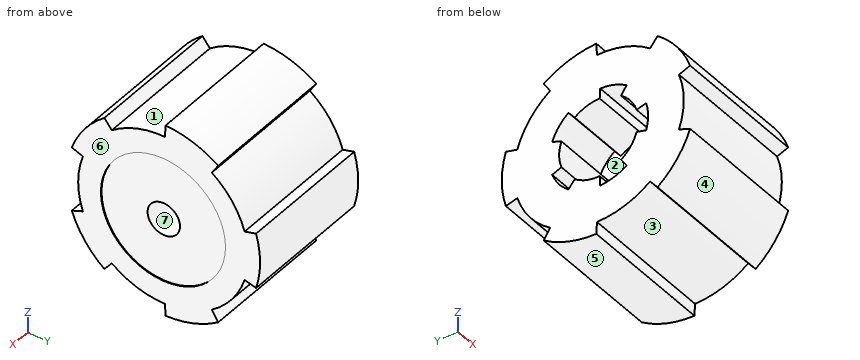
from build123d import *

# Parameters (mm, degrees)
SKETCH4_R                 = 21.5
BOSS_EXTRUDE1_DEPTH       = 34
BOSS_EXTRUDE2_DEPTH       = 34
CIRPATTERN1_COUNT         = 5
SKETCH7_R                 = 10
SHORTSHAFT_KEY1_DEPTH     = 16
SHORTSHAFT_KEY2_DEPTH     = 16
SHORTSHAFT_KEY_PATT_COUNT = 5
SKETCH10_R                = 15.75
PULLEYINDENTATION_DEPTH   = 0.2
SKETCH11_R                = 4.1
METAL_SHAFT_HOLE_DEPTH    = 14.5


with BuildPart() as part:
    # Sketch4 → Boss-Extrude1 (new body)
    with BuildSketch(Plane(origin=(0, 0, 0), x_dir=(0, 0, -1), z_dir=(1, 0, 0))):
        Circle(SKETCH4_R)
    extrude(amount=-BOSS_EXTRUDE1_DEPTH)

    # Sketch5 → Boss-Extrude2 (add)
    with BuildSketch(Plane(origin=(0, 0, 0), x_dir=(0, 0, -1), z_dir=(1, 0, 0))):
        with BuildLine():
            Line((-6.223542865, 20.579541156), (-7, 23.477318635))
            ThreePointArc((-7, 23.477318635), (0, 24.498663031), (7, 23.477318635))
            Line((7, 23.477318635), (6.223542865, 20.579541156))
            ThreePointArc((6.223542865, 20.579541156), (0, 21.5), (-6.223542865, 20.579541156))
        make_face()
    boss_extrude2 = extrude(amount=-BOSS_EXTRUDE2_DEPTH)

    # CirPattern1: Boss-Extrude2 ×5 about axis
    cirpattern1_axis = Axis((0, 0, 0), (1, 0, 0))
    for i in range(1, CIRPATTERN1_COUNT):
        add(boss_extrude2.rotate(cirpattern1_axis, i * 360 / CIRPATTERN1_COUNT))

    # Sketch7 → ShortShaft Key1 (cut)
    with BuildSketch(Plane.ZY.offset(34)):
        Circle(SKETCH7_R)
    extrude(amount=-SHORTSHAFT_KEY1_DEPTH, mode=Mode.SUBTRACT)

    # Sketch8 → ShortShaft Key2 (cut)
    with BuildSketch(Plane.ZY.offset(34)):
        with BuildLine():
            Line((-7.941654077, 6.077016581), (-9.88451898, 7.650317559))
            ThreePointArc((-9.88451898, 7.650317559), (-7.346870668, 10.11209996), (-4.22140002, 11.764814325))
            Line((-4.22140002, 11.764814325), (-3.325480146, 9.430863258))
            ThreePointArc((-3.325480146, 9.430863258), (-5.877852523, 8.090169944), (-7.941654077, 6.077016581))
        make_face()
    shortshaft_key2 = extrude(amount=-SHORTSHAFT_KEY2_DEPTH, mode=Mode.SUBTRACT)

    # ShortShaft Key Patt: ShortShaft Key2 ×5 about axis
    shortshaft_key_patt_axis = Axis((0, 0, 0), (1, 0, 0))
    for i in range(1, SHORTSHAFT_KEY_PATT_COUNT):
        add(shortshaft_key2.rotate(shortshaft_key_patt_axis, i * 360 / SHORTSHAFT_KEY_PATT_COUNT), mode=Mode.SUBTRACT)

    # Sketch10 → PulleyIndentation (cut)
    with BuildSketch(Plane(origin=(0, 0, 0), x_dir=(0, 0, -1), z_dir=(1, 0, 0))):
        Circle(SKETCH10_R)
    extrude(amount=-PULLEYINDENTATION_DEPTH, mode=Mode.SUBTRACT)

    # Sketch11 → Metal Shaft Hole (cut)
    with BuildSketch(Plane(origin=(0, 0, 0), x_dir=(0, 0, -1), z_dir=(1, 0, 0))):
        Circle(SKETCH11_R)
    extrude(amount=-METAL_SHAFT_HOLE_DEPTH, mode=Mode.SUBTRACT)


solid = part.part
For this review, take the finished solid that the model builds, in its own axes (mm). Face numbers are marked on the shaded views. A direction names the side the tool comes from. Give positions to 0.01 mm unless a question says otherwise; leave off trailing zeros. Write each loop counter-clockwise with the first axis right and the second up, starting at its lowest first coordinate (ties: lowest second). Pieces come first, ordered by that corner, then holes. Notation, with made-up numbers: (17.5, -29) -> (60.5, -29) arc R14 cw to (60.5, -22) -> close; hole circle Ø2 at (-29.5, -12). An arc over 180 degrees is marked (long way). Use CSV: the item, a comma, the result in double quotes.
Q1. Mouldability with a two-part tool opening along Y and no side actions: class the marked faces 4, 5, 6 and 7 as pulls with the +Y half, pulls with the -Y half, needs draft (parallel to the pull), parting line crosses it, or undercut.
Conclusion:
face 4,"pulls with the -Y half"
face 5,"pulls with the +Y half"
face 6,"needs draft"
face 7,"undercut"
Q2. To check wall thickness, follow probe 1 along X at (y, z) = (-13, -7.5); probe 2 along X at (y, z) = (6.5, -1); probe 3 along Y at (x, z) = (-23, 6) (3 decimals). State the ranges of each line that lie inside material, in increasing order. Write a range as [from, to].
Conclusion:
probe 1,"[-34, -0.2]"
probe 2,"[-18, -0.2]"
probe 3,"[-20.646, -8], [10.965, 23.753]"
Q3. Take a section at B-B, the plane z = 0. Write out the cut boundary in (x, y), then the cut area to 3 significant figures.
Conclusion:
outline,"(-34, -21.5) -> (0, -21.5) -> (0, -15.75) -> (-0.2, -15.75) -> (-0.2, -4.1) -> (-14.5, -4.1) -> (-14.5, 4.1) -> (-0.2, 4.1) -> (-0.2, 15.75) -> (0, 15.75) -> (0, 24.5) -> (-34, 24.5) -> (-34, 10) -> (-18, 10) -> (-18, -12.5) -> (-34, -12.5) -> close"
area,"1,080 mm2"
Q4. For P1, Ø6, axis at x = -14.5, y = 9, coming from the -Z side; P2, Ø7.5, axis at y = 0, z = 0, coming from the +X side; P3, Ø6, axis at x = -30, y = -4, coming from the -Z side, all flat-tipped, find the tip position at first contact; note any pin that passes through.
Conclusion:
P1,"z = -23.75"
P2,"x = -14.5"
P3,"z = -21.48"
Q5. Take a section at C-C, the plane y = -2. Write out the cut boundary in (x, z).
Conclusion:
outline,"(-34, -21.41) -> (0, -21.41) -> (0, -15.62) -> (-0.2, -15.62) -> (-0.2, -3.58) -> (-14.5, -3.58) -> (-14.5, 3.58) -> (-0.2, 3.58) -> (-0.2, 15.62) -> (0, 15.62) -> (0, 21.41) -> (-34, 21.41) -> (-34, 12.34) -> (-18, 12.34) -> (-18, -12.34) -> (-34, -12.34) -> close"
Q6. Take a section at D-D, the plane y = -17. Write out the cut boundary in (x, z), then the cut area to 3 significant figures.
Conclusion:
outline,"(-34, -17.64) -> (0, -17.64) -> (0, 17.64) -> (-34, 17.64) -> close"
area,"1,200 mm2"
Q7. Take a section at A-A, the plane x = -10. Write out the cut boundary in (y, z).
Conclusion:
outline,"(-23.11, -8.14) arc R24.5 ccw to (-14.88, -19.46) -> (-12.99, -17.13) arc R21.5 ccw to (0.44, -21.5) -> (0.6, -24.49) arc R24.5 ccw to (13.91, -20.17) -> (12.28, -17.65) arc R21.5 ccw to (20.58, -6.22) -> (23.48, -7) arc R24.5 ccw to (23.48, 7) -> (20.58, 6.22) arc R21.5 ccw to (12.28, 17.65) -> (13.91, 20.17) arc R24.5 ccw to (0.6, 24.49) -> (0.44, 21.5) arc R21.5 ccw to (-12.99, 17.13) -> (-14.88, 19.46) arc R24.5 ccw to (-23.11, 8.14) -> (-20.31, 7.06) arc R21.5 ccw to (-20.31, -7.06) -> close; hole circle Ø8.2 at (0, 0)"
Q8. Tool access review of the marked faces 1, 2 and 3: name each direction out of +Z, -Z, +X, -X, +Y, -Y from which nothing blocks a thin tool from reaching the whole face with its end or side.
Conclusion:
face 1,"+Z, +X, -X"
face 2,"-X"
face 3,"-Z, +X, -X"
